Can you work these out from the model? Positions are in its coordinate system, mm. Face numbers are marked on the shaded views. A direction names the side the tool comes from. Coordinates: 2 decimals unless noted, no trailing zeros. Order: outer loops, then holes, each group sorted by start corner. A loop starts at its lowest first (then second) coordinate and runs counter-clockwise, first axis right, second up. Notation, with made-up numbers: (89.25, -34) -> (111.25, -34) arc R19 ccw to (111.25, -22) -> close; hole circle Ø3 at (-22.5, 39). An arc over 180 degrees is marked (long way). Answer as CSV lines item,"result".
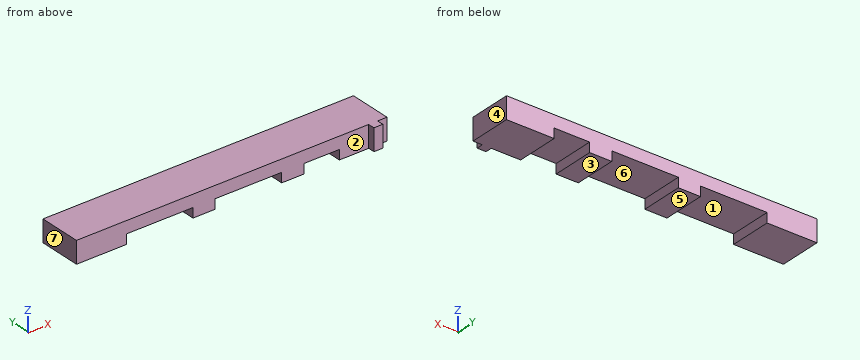
from build123d import *

# Parameters (mm, degrees)
SKETCH_1_W          = 4.9
SKETCH_1_H          = 9.6
EXTRUDE_1_DEPTH     = 70
SKETCH_2_W          = 8
SKETCH_2_H          = 2.159316865
SKETCH_2_W_2        = 15
CUT_EXTRUDE_1_DEPTH = 71.717892378
SKETCH_3_W          = 2
SKETCH_3_H          = 4.9
EXTRUDE_2_DEPTH     = 1.5


with BuildPart() as part:
    # 草图1 → 凸台-拉伸1 (new body)
    with BuildSketch(Plane(origin=(0, 0, 0), x_dir=(0, 0, -1), z_dir=(1, 0, 0))):
        with Locations((0.526626016, -3.550608051)):
            Rectangle(SKETCH_1_W, SKETCH_1_H)
    extrude(amount=EXTRUDE_1_DEPTH)

    # 草图2 → 切除-拉伸1 (cut, through all)
    with BuildSketch(Plane.XZ.offset(8.350608051)):
        with Locations((55.26, -1.896967583)):
            Rectangle(SKETCH_2_W, SKETCH_2_H)
        with Locations((38.76, -1.896967583)):
            Rectangle(SKETCH_2_W_2, SKETCH_2_H)
        with Locations((18.76, -1.896967583)):
            Rectangle(SKETCH_2_W_2, SKETCH_2_H)
    extrude(amount=-CUT_EXTRUDE_1_DEPTH, mode=Mode.SUBTRACT)

    # 草图3 → 凸台-拉伸2 (add)
    with BuildSketch(Plane.XZ.offset(8.350608051)):
        with Locations((66.88, -0.526626016)):
            Rectangle(SKETCH_3_W, SKETCH_3_H)
    extrude(amount=EXTRUDE_2_DEPTH)


solid = part.part
Q1. Imagine slicing it at C-C (y = -4.75). List the corners of the cut face in (x, z) for me.
Solution:
outline,"(0, -2.98) -> (11.26, -2.98) -> (11.26, -0.82) -> (26.26, -0.82) -> (26.26, -2.98) -> (31.26, -2.98) -> (31.26, -0.82) -> (46.26, -0.82) -> (46.26, -2.98) -> (51.26, -2.98) -> (51.26, -0.82) -> (59.26, -0.82) -> (59.26, -2.98) -> (70, -2.98) -> (70, 1.92) -> (0, 1.92) -> close"
Q2. Imagine slicing it at B-B (z = 0.7). List the corners of the cut face in (x, y) for me, and give its area (3 significant figures).
Solution:
outline,"(0, -8.35) -> (65.88, -8.35) -> (65.88, -9.85) -> (67.88, -9.85) -> (67.88, -8.35) -> (70, -8.35) -> (70, 1.25) -> (0, 1.25) -> close"
area,"675 mm2"
Q3. Imagine slicing it at D-D (x = 60.5). List the corners of the cut face in (y, z) for me.
Solution:
outline,"(-8.35, -2.98) -> (1.25, -2.98) -> (1.25, 1.92) -> (-8.35, 1.92) -> close"
Q4. If I drill on line 1 (X direction, y = -2.5, z = -1.35); line 2 (Z direction, x = 20, y = -1); line 3 (X direction, y = -8.5, z = -1), over which ranges is the centre line in solid material (lowest first)?
Solution:
line 1,"0 to 11.26, 26.26 to 31.26, 46.26 to 51.26, 59.26 to 70"
line 2,"-0.82 to 1.92"
line 3,"65.88 to 67.88"
Q5. For P1, Ø1.5, axis at x = 52.5, z = 0, coming from the -Y side; P2, Ø4, axis at x = 56.5, y = -2, coming from the -Z side; P3, Ø0.8, axis at y = -9, z = -1, coming from the -X side, each with a flat end and sliding along its axis, tell me the tip position at first contact or that it passes through.
Solution:
P1,"y = -8.35"
P2,"z = -0.82"
P3,"x = 65.88"
Q6. Which directions (+Z, -Z, +X, -X, +Y, -Y) give clear straight access to the entire face, cutting with the end or side of a thin tool? Please do the marked faces 1, 2 and 3.
Solution:
face 1,"-Z, +Y, -Y"
face 2,"+Z, -Z, -X, -Y"
face 3,"-Z, +X, -X, +Y, -Y"
Q7. We'd pull the mould along X, two halves only. Please class the marked faces 4, 5, 6 and 7: pulls with the +X half, pulls with the -X half, needs draft (parallel to the pull), parting line crosses it, or undercut.
Solution:
face 4,"pulls with the +X half"
face 5,"needs draft"
face 6,"undercut"
face 7,"pulls with the -X half"
Q8. Imagine slicing it at A-A (z = -2.3). List the corners of the cut face in (x, y) for me, and give its area (3 significant figures).
Solution:
outline,"(0, -8.35) -> (11.26, -8.35) -> (11.26, 1.25) -> (0, 1.25) -> close; (26.26, -8.35) -> (31.26, -8.35) -> (31.26, 1.25) -> (26.26, 1.25) -> close; (46.26, -8.35) -> (51.26, -8.35) -> (51.26, 1.25) -> (46.26, 1.25) -> close; (59.26, -8.35) -> (65.88, -8.35) -> (65.88, -9.85) -> (67.88, -9.85) -> (67.88, -8.35) -> (70, -8.35) -> (70, 1.25) -> (59.26, 1.25) -> close"
area,"310 mm2"
